Model file for the job. Use its own axes, mm. A direction names the side the tool comes from. Coordinates: 2 decimals unless noted, no trailing zeros. Write each loop counter-clockwise with the first axis right and the second up, starting at its lowest first coordinate (ties: lowest second). Pieces come first, ordered by that corner, then holes. Notation, with made-up numbers: M 57,-26 L 113,-26 A11 cw 113,-19 Z; hole C 11,60 d10. An arc over 180 degrees is marked long. One line per question, with ' | ' between items. Start each with the question number.
(1) Flat gauge pins, fed straight in: pin 1 Ø1 at (x, y) = (19, 17.5) entering from +Z; pin 2 Ø0.8 at (x, y) = (26.5, 6) entering from +Z; pin 3 Ø0.5 at (y, z) = (27.5, 8) entering from +X; pin 4 Ø1.5 at (x, z) = (16.5, 4.5) entering from -Y. Where does each tip first touch, or does it go through?
(2) Wall check: probe 1 along Y at (x, z) = (3.75, 7.25); probe 2 along Y at (x, z) = (24.5, 7.75). Give the ranges that are in metal, low to high.
(3) Cut at B-B (y = 15.25). Write the cut outline in (x, z), plus the area to 3 significant figures.
(4) Cut at A-A (z = 1.5). Write the cut outline in (x, y), plus the area to 3 significant figures.
(5) Tool access for faces 1 (the face through (8.67, 2.24, 3.23)), 2 (the face through (26.74, 9.785, 5.699)), 3 (the face through (14, 26, 2)): list every direction of +Z, -Z, +X, -X, +Y, -Y with a clear straight run to the whole face (end or side of a thin tool).
(6) Cut at D-D (z = 4.5). Write the cut outline in (x, y).
(7) Cut at C-C (x = 25.5). Write the cut outline in (y, z), plus the area to 3 significant figures.
(8) Two-plate mould, pull along X, no slides. Class faces 4 (the face through (29, 14, 1)), 5 (the face through (14, 15, 1)), 6 (the face through (2.24, 19.801, 3.285)), 7 (the face through (15, 27, 3)): +X half, -X half, draft (parallel to the pull), parting line (faces both ways), or undercut.
Autodesk Fusion 360 part; units mm, degrees
sketch "Skizze1" plane through (0, 0, 0) normal (0, 0, 1) x (1, 0, 0)
  line L0 (0, 0) -> (29, 0)
  line L1 (29, 0) -> (29, 29)
  line L2 (29, 29) -> (0, 29)
  line L3 (0, 29) -> (0, 0)
  dimension "d1" = 29
  dimension "d2" = 29
extrude "Extrusion1" add sketch "Skizze1" along normal blind 1
fillet "Abrundung1" radius 0.7 4 edges at (14.5, 0, 0) (29, 14.5, 0) (14.5, 29, 0) (0, 14.5, 0)
sketch "Skizze2" plane through (0, 0, 1) normal (0, 0, 1) x (-1, 0, 0)
  line L0 (0, -29) -> (0, 0)
  line L1 (0, 0) -> (-29, 0)
  line L2 (-29, 0) -> (-29, -29)
  line L3 (-29, -29) -> (0, -29)
  line L4 (-1.5, -27.5) -> (-27.5, -27.5)
  line L5 (-27.5, -27.5) -> (-27.5, -1.5)
  line L6 (-27.5, -1.5) -> (-1.5, -1.5)
  line L7 (-1.5, -1.5) -> (-1.5, -27.5)
  line L8 (-26, -26) -> (-26, -3)
  line L9 (-26, -3) -> (-3, -3)
  line L10 (-3, -3) -> (-3, -26)
  line L11 (-3, -26) -> (-26, -26)
  dimension "d7" = 26
  dimension "d8" = 26
  dimension "d9" = 29
  dimension "d10" = 1.5
  dimension "d11" = 1.5
  dimension "d12" = 1.5
extrude "Extrusion2" add sketch "Skizze2" along normal blind 2 contours L4 L5 L6 L7
sketch "Skizze3" plane through (1.5, 0, 0) normal (-1, 0, 0) x (0, -1, 0)
  line L0 (-27.5, 1) -> (-1.5, 1)
  line L1 (-1.5, 1) -> (-1.5, 3)
  line L2 (-1.5, 3) -> (-27.5, 3)
  line L3 (-27.5, 3) -> (-27.5, 1)
  line L4 (-9.5, 4) -> (-9.5, 5)
  line L5 (-10.5, 6) -> (-18.5, 6)
  line L6 (-19.5, 5) -> (-19.5, 4)
  line L7 (-8.5, 3) -> (-1.5, 3)
  line L8 (-27.5, 3) -> (-20.5, 3)
  arc A0 (-20.5, 3) -> (-19.5, 4) centre (-20.5, 4) ccw
  line L9 (-9.5, 3) -> (-1.5, 3)
  arc A1 (-9.5, 4) -> (-8.5, 3) centre (-8.5, 4) ccw
  arc A2 (-18.5, 6) -> (-19.5, 5) centre (-18.5, 5) ccw
  arc A3 (-9.5, 5) -> (-10.5, 6) centre (-10.5, 5) ccw
  point P0 (-19.5, 3)
  point P1 (-19.5, 6)
  dimension "d15" = 10
  dimension "d16" = 3
  dimension "d17" = 26
  dimension "d18" = 8
  dimension "d19" = 1
  dimension "d20" = 1
  dimension "d21" = 1
  dimension "d22" = 1
extrude "Extrusion3" add sketch "Skizze3" against normal up to surface (26 mm away) contours L2 L4 L5 L6 A0 L9 A1 A2 A3
extrude "Extrusion4" cut 1 faces at (10.6667, 18.3333, 1) along direction (0, 0, 1) blind 5
sketch "Skizze4" plane through (0, 27.5, 0) normal (0, 1, 0) x (-1, 0, 0)
  line L0 (-27.5, 1) -> (-1.5, 1)
  line L1 (-1.5, 1) -> (-1.5, 3)
  line L2 (-1.5, 3) -> (-27.5, 3)
  line L3 (-27.5, 3) -> (-27.5, 1)
sketch "Skizze5" plane through (0, 0, 1) normal (0, 0, 1) x (-1, 0, 0)
  line L0 (0, -29) -> (0, 0)
  line L1 (0, 0) -> (-29, 0)
  line L2 (-29, 0) -> (-29, -29)
  line L3 (-29, -29) -> (0, -29)
  line L4 (-1.5, -1.5) -> (-1.5, -27.5)
  line L5 (-1.5, -27.5) -> (-27.5, -27.5)
  line L6 (-27.5, -27.5) -> (-27.5, -1.5)
  line L7 (-27.5, -1.5) -> (-1.5, -1.5)
  line L8 (-27.5, -16.65) -> (-29, -16.65)
  line L9 (-29, -16.65) -> (-29, -12.35)
  line L10 (-29, -12.35) -> (-27.5, -12.35)
  line L11 (-27.5, -12.35) -> (-27.5, -16.65)
  line L12 (-27.5, -12.35) -> (0, -12.35) construction
  line L13 (0, -12.35) -> (-1.5, -12.35)
  line L14 (-1.5, -12.35) -> (-1.5, -16.65)
  line L15 (-1.5, -16.65) -> (0, -16.65)
  line L16 (0, -16.65) -> (0, -12.35)
  dimension "d27" = 4.3
  dimension "d28" = 29
  dimension "d29" = 12.35
  dimension "d30" = 4.3
extrude "Extrusion5" add sketch "Skizze5" along normal blind 1 contours L0 L4 L13 L14 L15 L16 | L2 L6 L8 L9 L10 L11
sketch "Skizze6" plane through (0, 27.5, 0) normal (0, 1, 0) x (-1, 0, 0)
  line L0 (-27.5, 1) -> (-1.5, 1)
  line L1 (-1.5, 1) -> (-1.5, 3)
  line L2 (-1.5, 3) -> (-27.5, 3)
  line L3 (-27.5, 3) -> (-27.5, 1)
  line L4 (-29.2103, 10) -> (4.3331, 10) construction
  line L5 (-1.5, 3) -> (-27.5, 3)
  line L6 (-1.5, 3) -> (-1.5, 10) construction
  line L7 (-1.5, 3) -> (-2, 10)
  line L8 (-14.5, 3) -> (-14.5, 12.4711) construction
  line L9 (-2, 10) -> (-6.1916, 10)
  line L10 (-7.1694, 9.2095) -> (-8.3306, 3.7905)
  line L11 (-1.5, 3) -> (-14.5, 3)
  arc A0 (-9.3084, 3) -> (-8.3306, 3.7905) centre (-9.3084, 4) ccw
  arc A1 (-6.1916, 10) -> (-7.1694, 9.2095) centre (-6.1916, 9) ccw
  line L12 (-21.8306, 9.2095) -> (-20.6694, 3.7905)
  arc A2 (-21.8306, 9.2095) -> (-22.8084, 10) centre (-22.8084, 9) ccw
  line L13 (-27, 10) -> (-22.8084, 10)
  line L14 (-27.5, 3) -> (-27, 10)
  arc A3 (-20.6694, 3.7905) -> (-19.6916, 3) centre (-19.6916, 4) ccw
  line L15 (-27.5, 3) -> (-14.5, 3)
  point P0 (-7, 10)
  dimension "d33" = 7
  dimension "d34" = 0.5
  dimension "d36" = 5
  dimension "d37" = 1
  dimension "d38" = 1
extrude "Extrusion6" add sketch "Skizze6" against normal up to surface (1.5 mm away) contours L2 L5 L12 A2 L13 L14 A3 L15 | L2 L5 L7 L9 L10 L11 A0 A1
sketch "Skizze7" plane through (27.5, 0, 0) normal (1, 0, 0) x (0, 1, 0)
  line L0 (16.65, 2) -> (16.65, 1)
  line L1 (16.65, 1) -> (27.5, 1)
  line L2 (27.5, 1) -> (27.5, 3)
  line L3 (27.5, 3) -> (26, 3)
  line L4 (26, 3) -> (20.5, 3)
  arc A0 (19.5, 4) -> (20.5, 3) centre (20.5, 4) ccw
  line L5 (19.5, 4) -> (19.5, 5)
  arc A1 (19.5, 5) -> (18.5, 6) centre (18.5, 5) ccw
  line L6 (18.5, 6) -> (10.5, 6)
  arc A2 (10.5, 6) -> (9.5, 5) centre (10.5, 5) ccw
  line L7 (9.5, 5) -> (9.5, 4)
  arc A3 (8.5, 3) -> (9.5, 4) centre (8.5, 4) ccw
  line L8 (8.5, 3) -> (1.5, 3)
  line L9 (1.5, 3) -> (1.5, 1)
  line L10 (1.5, 1) -> (12.35, 1)
  line L11 (12.35, 1) -> (12.35, 2)
  line L12 (12.35, 2) -> (16.65, 2)
  line L13 (26, 10) -> (26, 3)
  line L14 (26, 3) -> (27.5, 3)
  line L15 (27.5, 3) -> (27.5, 10)
  line L16 (27.5, 10) -> (26, 10)
  line L17 (26, 10) -> (27.6131, 8.3869)
  line L18 (26, 10) -> (28.2813, 10) construction
  dimension "d41" = 45
extrude "Extrusion7" cut sketch "Skizze7" against normal blind 29 contours L15 L16 L17
sketch "Skizze9" plane through (27.5, 0, 0) normal (1, 0, 0) x (0, 1, 0)
  line L0 (16.65, 2) -> (16.65, 1)
  line L1 (16.65, 1) -> (27.5, 1)
  line L2 (27.5, 1) -> (27.5, 3)
  line L3 (27.5, 3) -> (26, 3)
  line L4 (26, 3) -> (20.5, 3)
  arc A0 (19.5, 4) -> (20.5, 3) centre (20.5, 4) ccw
  line L5 (19.5, 4) -> (19.5, 5)
  arc A1 (19.5, 5) -> (18.5, 6) centre (18.5, 5) ccw
  line L6 (18.5, 6) -> (10.5, 6)
  arc A2 (10.5, 6) -> (9.5, 5) centre (10.5, 5) ccw
  line L7 (9.5, 5) -> (9.5, 4)
  arc A3 (8.5, 3) -> (9.5, 4) centre (8.5, 4) ccw
  line L8 (8.5, 3) -> (1.5, 3)
  line L9 (1.5, 3) -> (1.5, 1)
  line L10 (1.5, 1) -> (12.35, 1)
  line L11 (12.35, 1) -> (12.35, 2)
  line L12 (12.35, 2) -> (16.65, 2)
  line L13 (27.5, 8.5) -> (26, 10)
  line L14 (26, 10) -> (26, 3)
  line L15 (26, 3) -> (27.5, 3)
  line L16 (27.5, 3) -> (27.5, 8.5)
  line L17 (27.5, 8.5) -> (27.8536, 8.1464)
  arc A4 (27.5, 7.2929) -> (27.8536, 8.1464) centre (27.5, 7.7929) ccw
  dimension "d44" = 1
extrude "Extrusion8" add sketch "Skizze9" against normal up to surface (26 mm away) contours L16 L17 A4
sketch "Skizze10" plane through (0, 27.5, 0) normal (0, 1, 0) x (-1, 0, 0)
  line L0 (-21.4199, 7.2929) -> (-27.1934, 7.2929)
  line L1 (-27.1934, 7.2929) -> (-27.5, 3)
  line L2 (-27.5, 3) -> (-27.5, 1)
  line L3 (-27.5, 1) -> (-1.5, 1)
  line L4 (-1.5, 1) -> (-1.5, 3)
  line L5 (-1.5, 3) -> (-1.8066, 7.2929)
  line L6 (-1.8066, 7.2929) -> (-7.5801, 7.2929)
  line L7 (-7.5801, 7.2929) -> (-8.3306, 3.7905)
  arc A0 (-9.3084, 3) -> (-8.3306, 3.7905) centre (-9.3084, 4) ccw
  line L8 (-9.3084, 3) -> (-19.6916, 3)
  arc A1 (-20.6694, 3.7905) -> (-19.6916, 3) centre (-19.6916, 4) ccw
  line L9 (-20.6694, 3.7905) -> (-21.4199, 7.2929)
  line L10 (-7.3214, 8.5) -> (-7.1694, 9.2095)
  line L11 (-21.8306, 9.2095) -> (-21.6786, 8.5)
  line L12 (-27.1071, 8.5) -> (-27, 10)
  line L13 (-2, 10) -> (-1.8929, 8.5)
  line L14 (-1.8929, 8.5) -> (-1.8066, 7.2929)
  line L15 (-7.3214, 8.5) -> (-7.5801, 7.2929)
  line L16 (-27.1071, 8.5) -> (-27.1934, 7.2929)
  line L17 (-21.6786, 8.5) -> (-21.4199, 7.2929)
  line L18 (-1.5, 8.1464) -> (-1.5, 7.2929)
  line L19 (-1.5, 8.1464) -> (-27.5, 8.1464)
  line L20 (-27.5, 8.1464) -> (-27.5, 7.2929)
  line L21 (-27.5, 7.2929) -> (-27.1934, 7.2929)
  line L22 (-27.1934, 7.2929) -> (-21.4199, 7.2929)
  line L23 (-21.4199, 7.2929) -> (-7.5801, 7.2929)
  line L24 (-7.5801, 7.2929) -> (-1.8066, 7.2929)
  line L25 (-1.8066, 7.2929) -> (-1.5, 7.2929)
  line L26 (-27, 10) -> (-27.1071, 8.5)
  line L27 (-27.1071, 8.5) -> (-27.5, 8.5)
  line L28 (-27.5, 8.5) -> (-27.5, 8.1464)
  line L29 (-27.5, 8.1464) -> (-1.5, 8.1464)
  line L30 (-1.5, 8.1464) -> (-1.5, 8.5)
  line L31 (-1.5, 8.5) -> (-1.8929, 8.5)
  line L32 (-1.8929, 8.5) -> (-2, 10)
  line L33 (-2, 10) -> (-6.1916, 10)
  arc A2 (-6.1916, 10) -> (-7.1694, 9.2095) centre (-6.1916, 9) ccw
  line L34 (-7.1694, 9.2095) -> (-7.3214, 8.5)
  line L35 (-7.3214, 8.5) -> (-21.6786, 8.5)
  line L36 (-21.6786, 8.5) -> (-21.8306, 9.2095)
  arc A3 (-21.8306, 9.2095) -> (-22.8084, 10) centre (-22.8084, 9) ccw
  line L37 (-22.8084, 10) -> (-27, 10)
  line L38 (-27.5, 8.5) -> (-1.5, 8.5)
  line L39 (-1.5, 8.5) -> (-1.5, 7.2929)
  line L40 (-1.5, 7.2929) -> (-27.5, 7.2929)
  line L41 (-27.5, 7.2929) -> (-27.5, 8.5)
extrude "Extrusion9" cut sketch "Skizze10" along normal blind 1.5 contours L15 L17 L19 L23 L29 L40 | L16 L19 L20 L21 L29 L40 L41 | L15 L17 L19 L29 L35 L38 | L16 L19 L27 L28 L29 L38 L41 | L14 L18 L19 L25 L29 L39 L40 | L14 L19 L29 L30 L31 L38 L39
sketch "Skizze11" plane through (0, 0, 1) normal (0, 0, 1) x (-1, 0, 0)
  line L0 (-27.5, -16.65) -> (-29, -16.65)
  line L1 (-29, -16.65) -> (-29, -29)
  line L2 (-29, -29) -> (0, -29)
  line L3 (0, -29) -> (0, -16.65)
  line L4 (0, -16.65) -> (-1.5, -16.65)
  line L5 (-1.5, -16.65) -> (-1.5, -27.5)
  line L6 (-1.5, -27.5) -> (-27.5, -27.5)
  line L7 (-27.5, -27.5) -> (-27.5, -16.65)
  ellipse E0 centre (-7.473, -27.5) end of major axis (-7.473, -27) minor radius 0.1071 (-7.5801, -27.5) -> (-7.3972, -27.8536) ccw
  ellipse E1 centre (-21.527, -27.5) end of major axis (-21.527, -28) minor radius 0.1071 (-21.6028, -27.8536) -> (-21.4199, -27.5) ccw
  ellipse E2 centre (-27.1577, -27.5) end of major axis (-27.1577, -27) minor radius 0.0357 (-27.1934, -27.5) -> (-27.1324, -27.8536) ccw
  ellipse E3 centre (-1.8423, -27.5) end of major axis (-1.8423, -28) minor radius 0.0357 (-1.8676, -27.8536) -> (-1.8066, -27.5) ccw
  line L8 (-7.5801, -27.5) -> (-5.5801, -27.5)
  line L9 (-5.5801, -27.5) -> (-5.5801, -29)
  line L10 (-5.5801, -29) -> (-7.5801, -29)
  line L11 (-7.5801, -29) -> (-7.5801, -27.5)
  line L12 (-21.4199, -27.5) -> (-23.4199, -27.5)
  line L13 (-23.4199, -27.5) -> (-23.4199, -29)
  line L14 (-23.4199, -29) -> (-21.4199, -29)
  line L15 (-21.4199, -29) -> (-21.4199, -27.5)
  dimension "d49" = 2
  dimension "d50" = 2
extrude "Extrusion10" cut sketch "Skizze11" along normal blind 12 contours L2 L6 L12 L13 L14 L15 | L2 L6 L8 L9 L10 L11
sketch "Skizze12" plane through (0, 0, 1) normal (0, 0, 1) x (-1, 0, 0)
  line L0 (-3, -3) -> (-26, -3)
  line L1 (-26, -3) -> (-26, -26)
  line L2 (-26, -26) -> (-3, -26)
  line L3 (-3, -26) -> (-3, -3)
  line L4 (-26, -14.5) -> (1.3472, -14.5)
  line L5 (-26, -14.5) -> (-29.3311, -14.5)
  line L6 (-29, -12.35) -> (-27.5, -12.35)
  line L7 (-27.5, -12.35) -> (-27.5, -1.5)
  line L8 (-27.5, -1.5) -> (-1.5, -1.5)
  line L9 (-1.5, -1.5) -> (-1.5, -12.35)
  line L10 (-1.5, -12.35) -> (0, -12.35)
  line L11 (0, -12.35) -> (0, 0)
  line L12 (0, 0) -> (-29, 0)
  line L13 (-29, 0) -> (-29, -12.35)
  line L14 (-29, -12.35) -> (-29, -16.65)
  line L15 (0, -16.65) -> (0, -12.35)
  line L16 (0, -14.5) -> (-29, -14.5)
  line L17 (-29, -14.5) -> (-29, 0)
  line L18 (-29, 0) -> (0, 0)
  line L19 (0, 0) -> (0, -14.5)
extrude "Extrusion11" cut sketch "Skizze12" along normal blind 8 and the other way blind 3 contours L0 L1 L3 L4 L16 | L0 L1 L3 L4 L5 L6 L7 L8 L9 L10 L14 L15 L16 L17 L19 | L6 L7 L8 L9 L10 L11 L12 L13 L17 L18 L19
mirror "Spiegeln1" about plane through (26, 14.5, 1) normal (0, -1, 0) of bodies 1 merged
equation "d10 = ( d9 - d7 ) / 2"
equation "d11 = d10"
equation "d18 = ( d17 - d15 ) / 2"
equation "d29 = ( d28 - d27 ) / 2"
equation "d30 = d27"
Filled in:
1) pin 1: z = 1 | pin 2: z = 3 | pin 3: x = 27.16 | pin 4: through
2) probe 1: 1.5 to 3, 26 to 27.5 | probe 2: 1 to 3, 26 to 28
3) outline: M 0,0.7 A0.7 ccw 0.7,0 L 28.3,0 A0.7 ccw 29,0.7 L 29,2 L 27.5,2 L 27.5,6 L 26,6 L 26,1 L 3,1 L 3,6 L 1.5,6 L 1.5,2 L 0,2 Z | area: 46.8 mm²
4) outline: M 0,12.35 L 1.5,12.35 L 1.5,1.5 L 27.5,1.5 L 27.5,12.35 L 29,12.35 L 29,16.65 L 27.5,16.65 L 27.5,27.5 L 1.5,27.5 L 1.5,16.65 L 0,16.65 Z; hole M 3,3 L 26,3 L 26,26 L 3,26 Z | area: 160 mm²
5) face 1: +Z, +Y, -Y | face 2: +Z, +X, -X | face 3: +Z
6) outline: M 1.5,9.5 L 3,9.5 L 3,19.5 L 1.5,19.5 Z; M 1.61,1.5 L 8.18,1.5 L 8.18,3 L 1.61,3 Z; M 1.61,26 L 8.18,26 L 8.18,27.5 L 1.61,27.5 Z; M 20.82,1.5 L 27.39,1.5 L 27.39,3 L 20.82,3 Z; M 20.82,26 L 27.39,26 L 27.39,27.5 L 20.82,27.5 Z; M 26,9.5 L 27.5,9.5 L 27.5,19.5 L 26,19.5 Z
7) outline: M 0,0.7 A0.7 ccw 0.7,0 L 28.3,0 A0.7 ccw 29,0.7 L 29,1 L 27.5,1 L 27.5,7.29 A0.5 ccw 27.85,8.15 L 26,10 L 26,1 L 3,1 L 3,10 L 1.15,8.15 A0.5 ccw 1.5,7.29 L 1.5,1 L 0,1 Z | area: 54.4 mm²
8) face 4: +X half | face 5: undercut | face 6: draft | face 7: undercut
